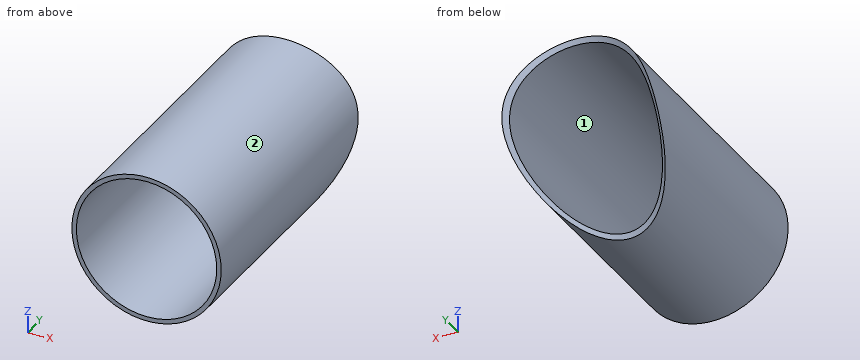
```python
from build123d import *

# Parameters (mm, degrees)
EXTRUDE_1_OUTLINE_R      = 50
EXTRUDE_1_OUTLINE_R_2    = 47
EXTRUDE_1_DEPTH          = 200
CUT_EXTRUDE_1_DEPTH      = 213.132034356
CUT_EXTRUDE_1_DEPTH_BACK = 213.132034356
SKETCH_2_R               = 66


# Read off the part's stored shape, not the designer's step: Вытянуть-Тонкостенный1
with BuildPart() as part:
    # Вытянуть-Тонкостенный1 outline → Вытянуть-Тонкостенный1 (new body)
    with BuildSketch(Plane(origin=(0, 0, 0), x_dir=(1, 0, 0), z_dir=(0, 1, 0))):
        Circle(EXTRUDE_1_OUTLINE_R)
        Circle(EXTRUDE_1_OUTLINE_R_2, mode=Mode.SUBTRACT)
    extrude(amount=EXTRUDE_1_DEPTH)

    # Эскиз2 → Вырез-Вытянуть1 (cut, two sides: drawn at the far end of the back side and taken through both)
    with BuildSketch(Plane(origin=(0, 0, 0), x_dir=(1, 0, 0), z_dir=(0, -0.5735764363510444, -0.819152044288993)).offset(-CUT_EXTRUDE_1_DEPTH_BACK)):
        with Locations((0, -180)):
            Circle(SKETCH_2_R)
    extrude(amount=CUT_EXTRUDE_1_DEPTH + CUT_EXTRUDE_1_DEPTH_BACK, mode=Mode.SUBTRACT)


solid = part.part
```
Can you work these out from the model? Positions are in its coordinate system, mm. Face numbers are marked on the shaded views. Coordinates: 2 decimals unless noted, no trailing zeros. Loops run counter-clockwise (first coordinate to the right, second up) from the corner with the lowest first, then second, coordinate; pieces in that order, holes last. Notation, with made-up numbers: (23.25, -10.75) - (40.25, -10.75) arc R13 ccw to (40.25, -2.75) - close; hole circle Ø11 at (-33.75, 51.25). An arc over 180 degrees is marked (long way). Answer as CSV lines item,"result". Start each with the question number.
1) Suppose I cut it at A-A (x = -25.5). Please give me the cut outline in (y, z), plus the area to 3 significant figures.
2) Thinking about a two-plate mould opening in X: for the marked faces 1 and 2, which applies, pulls with the +X half, pulls with the -X half, needs draft (parallel to the pull), parting line crosses it, or undercut?
3) I need wall thicknesses on line 1 (X direction, y = 108.5, z = 0); line 2 (Z direction, x = 33, y = 76.5). Which ranges of each line are inside material? Lowest first, please. Write a range as from..to.
4) For pin 1 (4 mm diameter, centred on y = 140, z = -20.5, fed in from -X); pin 2 (3 mm diameter, centred on x = -1.5, y = 138, fed in from -Z); pin 3 (1.5 mm diameter, centred on x = 21, y = 111.5, fed in from +Z), each with a flat end and sliding along its axis, tell me the tip position at first contact or that it passes through.
5) Suppose I cut it at C-C (x = -36). Please give me the cut outline in (y, z).
6) Suppose I cut it at B-B (y = 86.5). Please give me the cut outline in (x, z), plus the area to 3 significant figures.
Check result:
1,outline,"(0, -43.01) - (115.31, -43.01) - (117.78, -39.48) - (0, -39.48) - close; (0, 39.48) - (173.07, 39.48) - (175.54, 43.01) - (0, 43.01) - close"
1,area,"1,030 mm²"
2,face 1,"undercut"
2,face 2,"parting line crosses it"
3,line 1,"x = -50..-47, 47..50"
3,line 2,"z = -37.56..-33.47, 33.47..37.56"
4,pin 1,"stops at x = -46.45"
4,pin 2,"stops at z = 46.9"
4,pin 3,"stops at z = 45.72"
5,outline,"(0, -34.7) - (127.91, -34.7) - (131.05, -30.22) - (0, -30.22) - close; (0, 30.22) - (173.37, 30.22) - (176.51, 34.7) - (0, 34.7) - close"
6,outline,"circle Ø100 at (0, 0); hole circle Ø94 at (0, 0)"
6,area,"914 mm²"
